from build123d import *

# Parameters (mm, degrees)
BOSS_EXTRUDE1_DEPTH = 3
BOSS_EXTRUDE2_DEPTH = 16.5


with BuildPart() as part:
    # Sketch1 → Boss-Extrude1 (new body)
    with BuildSketch(Plane.XY):
        Polygon((0, 0), (91, -1.218180248), (91, -42), (66, -95.148154165), (0, -95.148154165), (0, -42), align=None)
    extrude(amount=BOSS_EXTRUDE1_DEPTH)

    # Sketch2 → Boss-Extrude2 (add)
    with BuildSketch(Plane.XY.offset(3)):
        Polygon((-2, -97.148154165), (67.269446555, -97.148154165), (93, -42.446897316), (93, 0.755225752), (-2, 2.026952385), align=None)
        Polygon((66, -95.148154165), (91, -42), (91, -1.218180248), (0, 0), (0, -95.148154165), align=None, mode=Mode.SUBTRACT)
    extrude(amount=-BOSS_EXTRUDE2_DEPTH)


solid = part.part
Geometry check sheet. Reference: the model listing, model coordinates, mm. A direction names the side the tool comes from. Round coordinates to 2 decimals unless told otherwise and drop trailing zeros. Order: outer loops, then holes, each group sorted by start corner. A loop starts at its lowest first (then second) coordinate and runs counter-clockwise, first axis right, second up. Notation, with made-up numbers: M 82.5,-31 L 91.5,-31 A21 cw 91.5,-2 Z; hole C -34.5,-3.75 d5. An arc over 180 degrees is marked long. Answer in a Markdown table with one row per item. Add a question column.
Item 1: Sectioned sample at C-C, the plane z = 1.5. Enter the section's corners in (x, y), plus the area to 3 significant figures.
Item 2: Set-up check for faces 5 (the face through (79.955, -70.18, -5.134)), 6 (the face through (46, -47, 0)): record each of +Z, -Z, +X, -X, +Y, -Y from which the full face is reachable in a straight line by a thin tool's end or side.
Item 3: Sectioned sample at A-A, the plane y = -7.5. Enter the section's corners in (x, z).
Item 4: Sectioned sample at D-D, the plane x = 63. Enter the section's corners in (y, z).
Item 5: Depth check by flat-ended pin: pin 1 Ø1.5 at (y, z) = (-76.5, 0) entering from +X; pin 2 Ø7 at (x, z) = (20.5, -4) entering from +Y; pin 3 Ø1.5 at (x, z) = (54.5, -3.5) entering from +Y. Enter the tip coordinate at first touch or a pass-through.
Item 6: Draft check along X on faces 1 (the face through (91, -22, -7)), 2 (the face through (-2, -47, -5)), 3 (the face through (38, 0, -13.5)), 4 (the face through (33, -95.148, -7)). Enter one of: released by +X, released by -X, zero draft, split by the parting line, or undercut.
Item 7: Sectioned sample at B-B, the plane z = -9.5. Enter the section's corners in (x, y), plus the area to 3 significant figures.
Item 8: Material ranges on L1, parallel to X at y = -36, z = -12; L2, parallel to Z at x = 16.5, y = -44; L3, parallel to Y at x = 55, z = -9, recorded low to high. Write a range as [from, to].
Filled in:
| question | item | result |
|---|---|---|
| 1 | outline | M -2,-97.15 L 67.27,-97.15 L 93,-42.45 L 93,0.76 L -2,2.03 Z |
| 1 | area | 8,660 mm² |
| 2 | face 5 | +Z, -Z, +X, -Y |
| 2 | face 6 | -Z |
| 3 | outline | M -2,-13.5 L 0,-13.5 L 0,0 L 91,0 L 91,-13.5 L 93,-13.5 L 93,3 L -2,3 Z |
| 4 | outline | M -97.15,-13.5 L -95.15,-13.5 L -95.15,0 L -0.84,0 L -0.84,-13.5 L 1.16,-13.5 L 1.16,3 L -97.15,3 Z |
| 5 | pin 1 | stops at x = 77.33 |
| 5 | pin 2 | stops at y = 1.77 |
| 5 | pin 3 | stops at y = 1.28 |
| 6 | face 1 | undercut |
| 6 | face 2 | released by -X |
| 6 | face 3 | zero draft |
| 6 | face 4 | undercut |
| 7 | outline | M -2,-97.15 L 67.27,-97.15 L 93,-42.45 L 93,0.76 L -2,2.03 Z; hole M 0,-95.15 L 66,-95.15 L 91,-42 L 91,-1.22 L 0,0 Z |
| 7 | area | 719 mm² |
| 8 | L1 | x = [-2, 0], [91, 93] |
| 8 | L2 | z = [0, 3] |
| 8 | L3 | y = [-97.15, -95.15], [-0.74, 1.26] |
